```python
from build123d import *
from OCP.BRepFilletAPI import BRepFilletAPI_MakeChamfer

# Parameters (mm, degrees)
ESTRUSIONE_ESTRUSIONE1_DEPTH                         = 66
RACCORDO1_R                                          = 10
SMUSSO1_SIZE                                         = 2
SMUSSO1_SIZE2                                        = 2.155800013
SMUSSO1_SIZE2_2                                      = 1.873732722
SMUSSO2_SIZE                                         = 5
FORO_LAMATO_PER_VITE_M4_A_TESTA_CILINDRI_D           = 4.5
FORO_LAMATO_PER_VITE_M4_A_TESTA_CILINDRI_DEPTH       = 30
FORO_LAMATO_PER_VITE_M4_A_TESTA_CILINDRI_CBORE_D     = 10
FORO_LAMATO_PER_VITE_M4_A_TESTA_CILINDRI_CBORE_DEPTH = 3
FORO_LAMATO_PER_VITE_M4_A_TESTA_CILINDRI_TIP         = 1.351936393
FORO_LAMATO_PER_VITE_M4_A_TESTA_CILI_2_D             = 4.5
FORO_LAMATO_PER_VITE_M4_A_TESTA_CILI_2_DEPTH         = 30
FORO_LAMATO_PER_VITE_M4_A_TESTA_CILI_2_CBORE_D       = 10
FORO_LAMATO_PER_VITE_M4_A_TESTA_CILI_2_CBORE_DEPTH   = 3
FORO_LAMATO_PER_VITE_M4_A_TESTA_CILI_2_TIP           = 1.351936393
FORO_LAMATO_PER_VITE_M4_A_TESTA_CILI_3_D             = 4.5
FORO_LAMATO_PER_VITE_M4_A_TESTA_CILI_3_DEPTH         = 45
FORO_LAMATO_PER_VITE_M4_A_TESTA_CILI_3_CBORE_D       = 10
FORO_LAMATO_PER_VITE_M4_A_TESTA_CILI_3_CBORE_DEPTH   = 32
FORO_LAMATO_PER_VITE_M4_A_TESTA_CILI_3_TIP           = 1.351936393


with BuildPart() as part:
    # Schizzo1 → Estrusione-Estrusione1 (new body)
    with BuildSketch(Plane.XY):
        Polygon((25.25, 100), (32.25, 100), (39.25, 0), (-39.25, 0), (-64.110342, 0), (-64.110342, 114.69), (-25.25, 114.69), (-25.25, 100), (-25.25, 15), (25.25, 15), align=None)
    extrude(amount=ESTRUSIONE_ESTRUSIONE1_DEPTH)

    # Raccordo1
    raccordo1_edges = [part.edges().sort_by_distance(p)[0] for p in [
        (-25.25, 15, 33),
        (25.25, 15, 33),
    ]]
    fillet(raccordo1_edges, radius=RACCORDO1_R)

    # Smusso1: one chamfer whose edges measure the first distance from different faces: ONE call of the kernel's chamfer builder (chamfer() names one face for all edges)
    smusso1_edges_1 = [part.edges().sort_by_distance(p)[0] for p in [
        (35.75, 50, 0),
        (-12.430171, 0, 0),
        (-64.110342, 57.345, 0),
        (-44.680171, 114.69, 0),
        (25.25, 62.5, 0),
        (25.25, 100, 33),
        (-44.680171, 114.69, 66),
        (-64.110342, 57.345, 66),
        (-12.430171, 0, 66),
        (-25.25, 69.845, 0),
        (-25.25, 69.845, 66),
        (0, 15, 0),
        (0, 15, 66),
        (-22.321067812, 17.928932188, 0),
        (-22.321067812, 17.928932188, 66),
        (35.75, 50, 66),
        (22.321067812, 17.928932188, 0),
        (22.321067812, 17.928932188, 66),
        (25.25, 62.5, 66),
    ]]
    smusso1_edges_2 = [part.edges().sort_by_distance(p)[0] for p in [
        (32.25, 100, 33),
    ]]
    smusso1_side_2 = [part.faces().sort_by_distance(p)[0] for p in [
        (35.75, 50, 33),
    ]]
    smusso1_edges_3 = [part.edges().sort_by_distance(p)[0] for p in [
        (39.25, 0, 33),
    ]]
    smusso1_side_3 = [part.faces().sort_by_distance(p)[0] for p in [
        (-12.430171, 0, 33),
    ]]
    smusso1 = BRepFilletAPI_MakeChamfer(part.part.solid().wrapped)
    for e in smusso1_edges_1:
        smusso1.Add(SMUSSO1_SIZE, e.wrapped)
    for e in smusso1_edges_2:
        smusso1.Add(SMUSSO1_SIZE, SMUSSO1_SIZE2, e.wrapped, smusso1_side_2[0].wrapped)  # the first distance lies on this face
    for e in smusso1_edges_3:
        smusso1.Add(SMUSSO1_SIZE, SMUSSO1_SIZE2_2, e.wrapped, smusso1_side_3[0].wrapped)  # the first distance lies on this face
    add(Compound.cast(smusso1.Shape()), mode=Mode.REPLACE)

    # Smusso2
    # the kernel refuses this chamfer: 5 mm, written as the material it takes off along each edge
    with BuildSketch(Plane(origin=(14.39158506, 100, 66), x_dir=(2.02935454733688e-15, -0.9996219169112968, 0.027495876610587663), z_dir=(1, 0, 0)), Plane(origin=(14.39158506, 100, 0), x_dir=(0, 0.0274958766105877, 0.9996219169112968), z_dir=(1, 0, 0))) as smusso2_piece_1:
        Polygon((SMUSSO2_SIZE * 0.999621916911, SMUSSO2_SIZE * 0.0274958766106), (-SMUSSO2_SIZE * 0.0274958766106, SMUSSO2_SIZE * 0.999621916911), (0, 0), align=None)
    extrude(amount=28.561029867, mode=Mode.SUBTRACT)

    # Foro lamato per Vite M4 a testa cilindri
    with Locations(Plane(origin=(35.25, 0, 0), x_dir=(0, 0, 1), z_dir=(1, 0, 0))):
        with Locations((56, -85.613628), (10, -85.613628)):
            CounterBoreHole(FORO_LAMATO_PER_VITE_M4_A_TESTA_CILINDRI_D / 2, FORO_LAMATO_PER_VITE_M4_A_TESTA_CILINDRI_CBORE_D / 2, FORO_LAMATO_PER_VITE_M4_A_TESTA_CILINDRI_CBORE_DEPTH, depth=FORO_LAMATO_PER_VITE_M4_A_TESTA_CILINDRI_DEPTH)
            with Locations((0, 0, -(FORO_LAMATO_PER_VITE_M4_A_TESTA_CILINDRI_DEPTH + FORO_LAMATO_PER_VITE_M4_A_TESTA_CILINDRI_TIP / 2))):  # 118° drill point
                Cone(0, FORO_LAMATO_PER_VITE_M4_A_TESTA_CILINDRI_D / 2, FORO_LAMATO_PER_VITE_M4_A_TESTA_CILINDRI_TIP, mode=Mode.SUBTRACT)

    # Foro lamato per Vite M4 a testa cili 2
    with Locations(Plane(origin=(0, 15, 0), x_dir=(1, 0, 0), z_dir=(0, 1, 0))):
        with Locations((-10.245584981, -33), (9.754415019, -33)):
            CounterBoreHole(FORO_LAMATO_PER_VITE_M4_A_TESTA_CILI_2_D / 2, FORO_LAMATO_PER_VITE_M4_A_TESTA_CILI_2_CBORE_D / 2, FORO_LAMATO_PER_VITE_M4_A_TESTA_CILI_2_CBORE_DEPTH, depth=FORO_LAMATO_PER_VITE_M4_A_TESTA_CILI_2_DEPTH)
            with Locations((0, 0, -(FORO_LAMATO_PER_VITE_M4_A_TESTA_CILI_2_DEPTH + FORO_LAMATO_PER_VITE_M4_A_TESTA_CILI_2_TIP / 2))):  # 118° drill point
                Cone(0, FORO_LAMATO_PER_VITE_M4_A_TESTA_CILI_2_D / 2, FORO_LAMATO_PER_VITE_M4_A_TESTA_CILI_2_TIP, mode=Mode.SUBTRACT)

    # Foro lamato per Vite M4 a testa cili 3
    with Locations(Plane.ZY.offset(64.110342)):
        with Locations((10, 85.613628), (56, 85.613628)):
            CounterBoreHole(FORO_LAMATO_PER_VITE_M4_A_TESTA_CILI_3_D / 2, FORO_LAMATO_PER_VITE_M4_A_TESTA_CILI_3_CBORE_D / 2, FORO_LAMATO_PER_VITE_M4_A_TESTA_CILI_3_CBORE_DEPTH, depth=FORO_LAMATO_PER_VITE_M4_A_TESTA_CILI_3_DEPTH)
            with Locations((0, 0, -(FORO_LAMATO_PER_VITE_M4_A_TESTA_CILI_3_DEPTH + FORO_LAMATO_PER_VITE_M4_A_TESTA_CILI_3_TIP / 2))):  # 118° drill point
                Cone(0, FORO_LAMATO_PER_VITE_M4_A_TESTA_CILI_3_D / 2, FORO_LAMATO_PER_VITE_M4_A_TESTA_CILI_3_TIP, mode=Mode.SUBTRACT)


solid = part.part
```
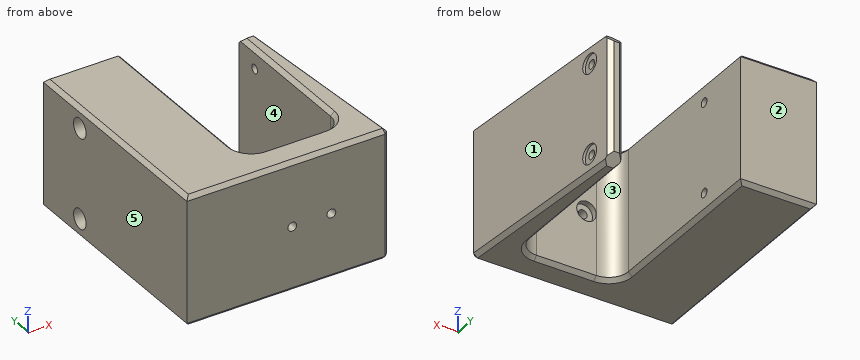
Verification items for the finished model (mm, model axes). Face numbers are marked on the shaded views. A direction names the side the tool comes from. Give positions to 0.01 mm unless a question says otherwise; leave off trailing zeros. Write each loop counter-clockwise with the first axis right and the second up, starting at its lowest first coordinate (ties: lowest second). Pieces come first, ordered by that corner, then holes. Notation, with made-up numbers: (-13, 86.5) - (27, 86.5) arc R16 ccw to (27, 100.5) - close; hole circle Ø4 at (-35, 29.5). An arc over 180 degrees is marked (long way). Put each result on its own line as item: value.
Q1. Section check C-C on y = 72.5. Record the cut outline in (x, z) (3 decimals), and give its area (3 significant figures).
Result:
outline: (-64.11, 2) - (-62.11, 0) - (-27.25, 0) - (-25.25, 2) - (-25.25, 64) - (-27.25, 66) - (-62.11, 66) - (-64.11, 64) - close; (25.25, 2) - (27.25, 0) - (32.17, 0) - (34.175, 2) - (34.175, 64) - (32.17, 66) - (27.25, 66) - (25.25, 64) - close
area: 3,140 mm2
Q2. Section check B-B on x = -9.5. Record the cut outline in (y, z).
Result:
outline: (0, 2) - (2, 0) - (13, 0) - (15, 2) - (15, 28.06) - (12, 28.06) - (12, 30.88) - (0, 30.88) - close; (0, 35.12) - (12, 35.12) - (12, 37.94) - (15, 37.94) - (15, 64) - (13, 66) - (2, 66) - (0, 64) - close
Q3. Set-up check for the marked faces 4 and 5: record each of +Z, -Z, +X, -X, +Y, -Y from which the full face is reachable in a straight line by a thin tool's end or side.
Result:
face 4: +Z, -Z, +Y
face 5: +Z, -Z, -X, +Y, -Y
Q4. Section check D-D on x = -42.5. Record the cut outline in (y, z).
Result:
outline: (0, 2) - (2, 0) - (112.69, 0) - (114.69, 2) - (114.69, 64) - (112.69, 66) - (2, 66) - (0, 64) - close; hole circle Ø10 at (85.61, 10); hole circle Ø10 at (85.61, 56)
Q5. Mould release check, pull along X, two halves, no side actions. Record for the marked faces 1, 2 and 3: released by +X, released by -X, zero draft, split by the parting line, or undercut.
Result:
face 1: released by +X
face 2: zero draft
face 3: undercut
Q6. Section check A-A on z = 33. Count the separate pieces of the cut face and the enclosed holes in it, and give its area (3 significant figures).
Result:
separate pieces: 3
enclosed holes: 0
area: 6,130 mm2
Q7. Depth check by flat-ended pin: P1, Ø8, axis at y = 22.5, z = 24.5, coming from the +X side (3 decimals); P2, Ø6, axis at x = -10.25, z = 33, coming from the -Y side; P3, Ø8, axis at y = 86, z = 54.5, coming from the +X side; P4, Ø1.4, axis at x = 29, z = 21.5, coming from the +Y side. Enter the tip coordinate at first touch or a pass-through.
Result:
P1: x = 37.955
P2: y = 0
P3: x = 33.42
P4: y = 100
Q8. Scan lines: probe 1 along Y at (x, z) = (-37.5, 56); probe 2 along Y at (x, z) = (-27.75, 10); probe 3 along X at (y, z) = (13, 36). Record each from-to range of solid material in increasing order. Write a range as from..to.
Result:
probe 1: 0..80.61, 90.61..114.69
probe 2: 0..83.36, 87.86..114.69
probe 3: -64.11..-14.25, -6.25..5.75, 13.75..38.34
